Autodesk Inventor part; units mm, degrees
ref_plane "YZ Plane" through (0, 0, 0) normal (1, 0, 0) x (0, 1, 0)
ref_plane "XZ Plane" through (0, 0, 0) normal (0, 1, 0) x (-1, 0, 0)
ref_plane "XY Plane" through (0, 0, 0) normal (0, 0, 1) x (1, 0, 0)
sketch "Sketch1" plane through (0, 0, 0) normal (0, 0, 1) x (1, 0, 0)
  circle A0 centre (0, 0) radius 3.925
  circle A1 centre (0, 0) radius 2
  dimension "d0" = 7.85
  dimension "d1" = 4
extrude "Extrusion1" add sketch "Sketch1" along normal blind 7
sketch "Sketch2" plane through (0, 0, 7) normal (0, 0, 1) x (1, 0, 0)
  circle A0 centre (0, 0) radius 8.75
  circle A1 centre (0, 0) radius 2
  dimension "d4" = 17.5
extrude "Extrusion2" add sketch "Sketch2" along normal blind 3.81
fillet "Fillet1" radius 3.175 1 edges at (-8.75, 0, 10.81)
properties part number "ball bearing connector"
Can you work these out from the model? Positions are in its coordinate system, mm. A direction names the side the tool comes from. Give positions to 0.01 mm unless a question says otherwise; leave off trailing zeros. Order: outer loops, then holes, each group sorted by start corner. A loop starts at its lowest first (then second) coordinate and runs counter-clockwise, first axis right, second up. Notation, with made-up numbers: M 10.5,56.5 L 29.5,56.5 A23 ccw 29.5,72.5 Z; hole C 79,-5 d7. An arc over 180 degrees is marked long. One line per item, written item: value.
1) On a 3-axis mill with a long thin cutter (end or side, diameter ignored), from which of +Z, -Z, +X, -X, +Y, -Y can I reach the whole of each face in a straight line? I mean faces 1 (the face through (-2, 1, 0)), 2 (the face through (-2.893, -2.653, 3.451)). Say none if no direction works.
Answer sheet:
face 1: -Z, +X, -X, +Y, -Y
face 2: -Z
2) I want a section at A-A, the plane x = 0. List the corners of the cut face in (y, z) for me (3 decimals), plus the area to 3 significant figures.
Answer sheet:
outline: M -8.75,7 L -3.925,7 L -3.925,0 L -2,0 L -2,10.81 L -5.575,10.81 A3.175 ccw -8.75,7.635 Z; M 2,0 L 3.925,0 L 3.925,7 L 8.75,7 L 8.75,7.635 A3.175 ccw 5.575,10.81 L 2,10.81 Z
area: 74.1 mm^2
3) For P1, Ø6, axis at x = 6, z = 8.5, coming from the +Y side, with a flat end and sliding along its axis, tell me the tip position at first contact or that it passes through.
Answer sheet:
P1: stops at y = 8.19
4) We'd pull the mould along Y, two halves only. Please class faces 3 (the face through (-6.944, 5.324, 7.313)), 4 (the face through (0, 2, 5)), 5 (the face through (2, -4, 7)): released by +Y, released by -Y, zero draft, split by the parting line, or undercut.
Answer sheet:
face 3: split by the parting line
face 4: undercut
face 5: zero draft
5) I want a section at D-D, the plane z = 8.5. List the corners of the cut face in (x, y) for me, plus the area to 3 significant figures.
Answer sheet:
outline: C 0,0 d17.26; hole C 0,0 d4
area: 221 mm^2
6) I want a section at C-C, the plane z = 4.25. List the corners of the cut face in (x, y) for me (3 decimals), plus the area to 3 significant figures.
Answer sheet:
outline: C 0,0 d7.85; hole C 0,0 d4
area: 35.8 mm^2
7) Please list where these lines run through material, in increasing order: line 1 along Y through (x, z) = (0, 3.75) (3 decimals); line 2 along Y through (x, z) = (-1.25, 9); line 3 along Z through (x, y) = (-1.5, -5.5).
Answer sheet:
line 1: y = -3.925 to -2, 2 to 3.925
line 2: y = -8.35 to -1.56, 1.56 to 8.35
line 3: z = 7 to 10.81
